Autodesk Inventor part; units mm, degrees
ref_plane "YZ Plane" through (0, 0, 0) normal (1, 0, 0) x (0, 1, 0)
ref_plane "XZ Plane" through (0, 0, 0) normal (0, 1, 0) x (-1, 0, 0)
ref_plane "XY Plane" through (0, 0, 0) normal (0, 0, 1) x (1, 0, 0)
sketch "Sketch1" plane through (0, 0, 0) normal (0, 0, 1) x (1, 0, 0)
  circle A0 centre (0, 0) radius 17.25
  circle A1 centre (0, 0) radius 16.1
  circle A2 centre (0, 0) radius 15
  line L0 (-1, -15.03) -> (1, -15.03)
  line L1 (-1.5, -16.03) -> (1.5, -16.03)
  line L2 (1.5, -16.03) -> (1, -15.03)
  line L3 (-1.5, -16.03) -> (-1, -15.03)
  line L4 (-1, -15.03) -> (-0.9693, -14.9686)
  line L5 (1, -15.03) -> (0.9693, -14.9686)
  line L6 (2.9241, -14.7767) -> (4.856, -14.259)
  line L7 (2.7, -15.872) -> (2.9241, -14.7767)
  line L8 (2.9241, -14.7767) -> (2.9379, -14.7095)
  line L9 (5.5978, -15.0955) -> (4.856, -14.259)
  line L10 (4.856, -14.259) -> (4.8105, -14.2077)
  line L11 (6.649, -13.5163) -> (8.381, -12.5163)
  line L12 (6.7159, -14.6324) -> (6.649, -13.5163)
  line L13 (6.649, -13.5163) -> (6.6449, -13.4479)
  line L14 (9.314, -13.1324) -> (8.381, -12.5163)
  line L15 (8.381, -12.5163) -> (8.3238, -12.4786)
  line L16 (9.9207, -11.3349) -> (11.3349, -9.9207)
  line L17 (10.2742, -12.3956) -> (9.9207, -11.3349)
  line L18 (9.9207, -11.3349) -> (9.899, -11.2699)
  line L19 (12.3956, -10.2742) -> (11.3349, -9.9207)
  line L20 (11.3349, -9.9207) -> (11.2699, -9.899)
  line L21 (12.5163, -8.381) -> (13.5163, -6.649)
  line L22 (13.1324, -9.314) -> (12.5163, -8.381)
  line L23 (12.5163, -8.381) -> (12.4786, -8.3238)
  line L24 (14.6324, -6.7159) -> (13.5163, -6.649)
  line L25 (13.5163, -6.649) -> (13.4479, -6.6449)
  line L26 (14.259, -4.856) -> (14.7767, -2.9241)
  line L27 (15.0955, -5.5978) -> (14.259, -4.856)
  line L28 (14.259, -4.856) -> (14.2077, -4.8105)
  line L29 (15.872, -2.7) -> (14.7767, -2.9241)
  line L30 (14.7767, -2.9241) -> (14.7095, -2.9379)
  line L31 (15.03, -1) -> (15.03, 1)
  line L32 (16.03, -1.5) -> (15.03, -1)
  line L33 (15.03, -1) -> (14.9686, -0.9693)
  line L34 (16.03, 1.5) -> (15.03, 1)
  line L35 (15.03, 1) -> (14.9686, 0.9693)
  line L36 (14.7767, 2.9241) -> (14.259, 4.856)
  line L37 (15.872, 2.7) -> (14.7767, 2.9241)
  line L38 (14.7767, 2.9241) -> (14.7095, 2.9379)
  line L39 (15.0955, 5.5978) -> (14.259, 4.856)
  line L40 (14.259, 4.856) -> (14.2077, 4.8105)
  line L41 (13.5163, 6.649) -> (12.5163, 8.381)
  line L42 (14.6324, 6.7159) -> (13.5163, 6.649)
  line L43 (13.5163, 6.649) -> (13.4479, 6.6449)
  line L44 (13.1324, 9.314) -> (12.5163, 8.381)
  line L45 (12.5163, 8.381) -> (12.4786, 8.3238)
  line L46 (11.3349, 9.9207) -> (9.9207, 11.3349)
  line L47 (12.3956, 10.2742) -> (11.3349, 9.9207)
  line L48 (11.3349, 9.9207) -> (11.2699, 9.899)
  line L49 (10.2742, 12.3956) -> (9.9207, 11.3349)
  line L50 (9.9207, 11.3349) -> (9.899, 11.2699)
  line L51 (8.381, 12.5163) -> (6.649, 13.5163)
  line L52 (9.314, 13.1324) -> (8.381, 12.5163)
  line L53 (8.381, 12.5163) -> (8.3238, 12.4786)
  line L54 (6.7159, 14.6324) -> (6.649, 13.5163)
  line L55 (6.649, 13.5163) -> (6.6449, 13.4479)
  line L56 (4.856, 14.259) -> (2.9241, 14.7767)
  line L57 (5.5978, 15.0955) -> (4.856, 14.259)
  line L58 (4.856, 14.259) -> (4.8105, 14.2077)
  line L59 (2.7, 15.872) -> (2.9241, 14.7767)
  line L60 (2.9241, 14.7767) -> (2.9379, 14.7095)
  line L61 (1, 15.03) -> (-1, 15.03)
  line L62 (1.5, 16.03) -> (1, 15.03)
  line L63 (1, 15.03) -> (0.9693, 14.9686)
  line L64 (-1.5, 16.03) -> (-1, 15.03)
  line L65 (-1, 15.03) -> (-0.9693, 14.9686)
  line L66 (-2.9241, 14.7767) -> (-4.856, 14.259)
  line L67 (-2.7, 15.872) -> (-2.9241, 14.7767)
  line L68 (-2.9241, 14.7767) -> (-2.9379, 14.7095)
  line L69 (-5.5978, 15.0955) -> (-4.856, 14.259)
  line L70 (-4.856, 14.259) -> (-4.8105, 14.2077)
  line L71 (-6.649, 13.5163) -> (-8.381, 12.5163)
  line L72 (-6.7159, 14.6324) -> (-6.649, 13.5163)
  line L73 (-6.649, 13.5163) -> (-6.6449, 13.4479)
  line L74 (-9.314, 13.1324) -> (-8.381, 12.5163)
  line L75 (-8.381, 12.5163) -> (-8.3238, 12.4786)
  line L76 (-9.9207, 11.3349) -> (-11.3349, 9.9207)
  line L77 (-10.2742, 12.3956) -> (-9.9207, 11.3349)
  line L78 (-9.9207, 11.3349) -> (-9.899, 11.2699)
  line L79 (-12.3956, 10.2742) -> (-11.3349, 9.9207)
  line L80 (-11.3349, 9.9207) -> (-11.2699, 9.899)
  line L81 (-12.5163, 8.381) -> (-13.5163, 6.649)
  line L82 (-13.1324, 9.314) -> (-12.5163, 8.381)
  line L83 (-12.5163, 8.381) -> (-12.4786, 8.3238)
  line L84 (-14.6324, 6.7159) -> (-13.5163, 6.649)
  line L85 (-13.5163, 6.649) -> (-13.4479, 6.6449)
  line L86 (-14.259, 4.856) -> (-14.7767, 2.9241)
  line L87 (-15.0955, 5.5978) -> (-14.259, 4.856)
  line L88 (-14.259, 4.856) -> (-14.2077, 4.8105)
  line L89 (-15.872, 2.7) -> (-14.7767, 2.9241)
  line L90 (-14.7767, 2.9241) -> (-14.7095, 2.9379)
  line L91 (-15.03, 1) -> (-15.03, -1)
  line L92 (-16.03, 1.5) -> (-15.03, 1)
  line L93 (-15.03, 1) -> (-14.9686, 0.9693)
  line L94 (-16.03, -1.5) -> (-15.03, -1)
  line L95 (-15.03, -1) -> (-14.9686, -0.9693)
  line L96 (-14.7767, -2.9241) -> (-14.259, -4.856)
  line L97 (-15.872, -2.7) -> (-14.7767, -2.9241)
  line L98 (-14.7767, -2.9241) -> (-14.7095, -2.9379)
  line L99 (-15.0955, -5.5978) -> (-14.259, -4.856)
  line L100 (-14.259, -4.856) -> (-14.2077, -4.8105)
  line L101 (-13.5163, -6.649) -> (-12.5163, -8.381)
  line L102 (-14.6324, -6.7159) -> (-13.5163, -6.649)
  line L103 (-13.5163, -6.649) -> (-13.4479, -6.6449)
  line L104 (-13.1324, -9.314) -> (-12.5163, -8.381)
  line L105 (-12.5163, -8.381) -> (-12.4786, -8.3238)
  line L106 (-11.3349, -9.9207) -> (-9.9207, -11.3349)
  line L107 (-12.3956, -10.2742) -> (-11.3349, -9.9207)
  line L108 (-11.3349, -9.9207) -> (-11.2699, -9.899)
  line L109 (-10.2742, -12.3956) -> (-9.9207, -11.3349)
  line L110 (-9.9207, -11.3349) -> (-9.899, -11.2699)
  line L111 (-8.381, -12.5163) -> (-6.649, -13.5163)
  line L112 (-9.314, -13.1324) -> (-8.381, -12.5163)
  line L113 (-8.381, -12.5163) -> (-8.3238, -12.4786)
  line L114 (-6.7159, -14.6324) -> (-6.649, -13.5163)
  line L115 (-6.649, -13.5163) -> (-6.6449, -13.4479)
  line L116 (-4.856, -14.259) -> (-2.9241, -14.7767)
  line L117 (-5.5978, -15.0955) -> (-4.856, -14.259)
  line L118 (-4.856, -14.259) -> (-4.8105, -14.2077)
  line L119 (-2.7, -15.872) -> (-2.9241, -14.7767)
  line L120 (-2.9241, -14.7767) -> (-2.9379, -14.7095)
  point P0 (0, -16.03)
  point P1 (0, -15.03)
  point P2 (1.5, -16.03)
  point P3 (1.5, -16.03)
  point P4 (3.89, -14.5178)
  point P5 (7.515, -13.0163)
  point P6 (10.6278, -10.6278)
  point P7 (13.0163, -7.515)
  point P8 (14.5178, -3.89)
  point P9 (15.03, 0)
  point P10 (14.5178, 3.89)
  point P11 (13.0163, 7.515)
  point P12 (10.6278, 10.6278)
  point P13 (7.515, 13.0163)
  point P14 (3.89, 14.5178)
  point P15 (0, 15.03)
  point P16 (-3.89, 14.5178)
  point P17 (-7.515, 13.0163)
  point P18 (-10.6278, 10.6278)
  point P19 (-13.0163, 7.515)
  point P20 (-14.5178, 3.89)
  point P21 (-15.03, 0)
  point P22 (-14.5178, -3.89)
  point P23 (-13.0163, -7.515)
  point P24 (-10.6278, -10.6278)
  point P25 (-7.515, -13.0163)
  point P26 (-3.89, -14.5178)
  point P27 (2.7, -15.872)
  point P28 (5.5978, -15.0955)
  point P29 (6.7159, -14.6324)
  point P30 (9.314, -13.1324)
  point P31 (10.2742, -12.3956)
  point P32 (12.3956, -10.2742)
  point P33 (14.6324, -6.7159)
  point P34 (15.872, -2.7)
  point P35 (16.03, -1.5)
  point P36 (16.03, 1.5)
  point P37 (15.872, 2.7)
  point P38 (15.0955, 5.5978)
  point P39 (14.6324, 6.7159)
  point P40 (13.1324, 9.314)
  point P41 (12.3956, 10.2742)
  point P42 (10.2742, 12.3956)
  point P43 (6.7159, 14.6324)
  point P44 (2.7, 15.872)
  point P45 (1.5, 16.03)
  point P46 (-1.5, 16.03)
  point P47 (-5.5978, 15.0955)
  point P48 (-6.7159, 14.6324)
  point P49 (-10.2742, 12.3956)
  point P50 (-12.3956, 10.2742)
  point P51 (-14.6324, 6.7159)
  point P52 (-15.0955, 5.5978)
  point P53 (-15.872, 2.7)
  point P54 (-16.03, -1.5)
  point P55 (-14.6324, -6.7159)
  point P56 (-12.3956, -10.2742)
  point P57 (-10.2742, -12.3956)
  point P58 (-9.314, -13.1324)
  point P59 (-6.7159, -14.6324)
  point P60 (-5.5978, -15.0955)
  point P61 (-2.7, -15.872)
  dimension "d1" = 32.2
  dimension "d0" = 34.5
  dimension "d2" = 30
  dimension "d3" = 2
  dimension "d4" = 3
  dimension "d5" = 1
  dimension "d20" = 360
extrude "Extrusion1" add sketch "Sketch1" along normal blind 15 contours L34 L35 A2 L38 L37 A1 | A1 L29 L30 A2 L33 L32 | L31 L33 A2 L35 | L39 L40 A2 L43 L42 A1 | L38 A2 L40 L36 | A2 | A1 L24 L25 A2 L28 L27 | L26 L28 A2 L30 | L44 L45 A2 L48 L47 A1 | L43 A2 L45 L41 | A1 L19 L20 A2 L23 L22 | L21 L23 A2 L25 | L49 L50 A2 L53 L52 A1 | L48 A2 L50 L46 | A1 L14 L15 A2 L18 L17 | L16 L18 A2 L20 | L54 L55 A2 L58 L57 A1 | L53 A2 L55 L51 | A1 L9 L10 A2 L13 L12 | L11 L13 A2 L15 | L59 L60 A2 L63 L62 A1 | L58 A2 L60 L56 | A1 L2 L5 A2 L8 L7 | L6 L8 A2 L10 | L64 L65 A2 L68 L67 A1 | L63 A2 L65 L61 | A1 L119 L120 A2 L4 L3 | L69 L70 A2 L73 L72 A1 | L68 A2 L70 L66 | A1 L114 L115 A2 L118 L117 | L116 L118 A2 L120 | L74 L75 A2 L78 L77 A1 | L73 A2 L75 L71 | A1 L109 L110 A2 L113 L112 | L111 L113 A2 L115 | L79 L80 A2 L83 L82 A1 | L78 A2 L80 L76 | A1 L104 L105 A2 L108 L107 | L106 L108 A2 L110 | L84 L85 A2 L88 L87 A1 | L83 A2 L85 L81 | A1 L99 L100 A2 L103 L102 | L101 L103 A2 L105 | L89 L90 A2 L93 L92 A1 | L88 A2 L90 L86 | A1 L94 L95 A2 L98 L97 | L96 L98 A2 L100 | L93 A2 L95 L91
sketch "Sketch2" plane through (0, 0, 0) normal (0, 0, -1) x (-1, 0, 0)
  line L0 (12, 6.9282) -> (12, -6.9282)
  line L1 (12, -6.9282) -> (0, -13.8564)
  line L2 (0, -13.8564) -> (-12, -6.9282)
  line L3 (-12, -6.9282) -> (-12, 6.9282)
  line L4 (-12, 6.9282) -> (0, 13.8564)
  line L5 (0, 13.8564) -> (12, 6.9282)
  point P0 (0, 0)
  point P1 (0, 0)
  dimension "d12" = 24
extrude "Extrusion2" add sketch "Sketch2" along normal blind 10
sketch "Sketch3" plane through (0, 0, -10) normal (0, 0, -1) x (-1, 0, 0)
  circle A0 centre (0, 0) radius 7.5
  dimension "d15" = 15
extrude "Extrusion3" [suppressed]
sketch "Sketch4" plane through (0, 0, 0) normal (1, 0, 0) x (0, 1, 0)
  line L0 (20.1089, -13.3141) -> (-23.1689, -13.3141)
  line L1 (-23.1689, -13.3141) -> (-23.1689, 5.9253)
  line L2 (-23.1689, 5.9253) -> (20.1089, 5.9253)
  line L3 (20.1089, 5.9253) -> (20.1089, -13.3141)
  point P0 (0, 0)
extrude "Extrusion4" [suppressed]
properties part number "Nastavek Millard freewheel tool izmerjen trapze"
Check sheet for the modelled part. Datum: model origin and axes. Units: mm. A direction names the side the tool comes from. Give positions to 0.01 mm unless a question says otherwise; leave off trailing zeros. Order: outer loops, then holes, each group sorted by start corner. A loop starts at its lowest first (then second) coordinate and runs counter-clockwise, first axis right, second up. Notation, with made-up numbers: M 41,56.25 L 77,56.25 A13 ccw 77,69.25 Z; hole C -27.75,25.25 d6. An arc over 180 degrees is marked long. Answer as CSV lines item,"result". Start each with the question number.
Item 1: Tool access check on faces 4 (the face through (2.11, -15.96, 7.4)), 5 (the face through (-15.33, -2.81, 7.4)), 6 (the face through (15.537, -1.253, 7.395)), 7 (the face through (-11.87, 10.1, 7.4)), 8 (the face through (8.854, -12.829, 7.395)). Record the directions out of +Z, -Z, +X, -X, +Y, -Y that give a thin tool (end or side, any length) a straight path to the whole face; none if there is none.
Item 2: Thickness scan on line 1 (Y direction, x = 13, z = 13); line 2 (X direction, y = -1, z = -1.75); line 3 (Z direction, x = -2.5, y = -13.5). Record the ranges inside material, lowest first. Write a range as [from, to].
Item 3: Gauge pin test, flat ends, axial feed: P1, Ø3, axis at y = -3, z = -3.5, coming from the +X side; P2, Ø2, axis at x = 9, y = -11, coming from the -Z side; P3, Ø1.5, axis at y = -8, z = 3.5, coming from the +X side; P4, Ø5, axis at x = -3.5, z = 3, coming from the +Y side. Record the tip position at first contact, or that the pin passes through.
Item 4: Cross-section at C-C on y = 2. Enter the section's corners in (x, z).
Item 5: Mould release check, pull along X, two halves, no side actions. Record for faces 1 (the face through (6.683, 14.082, 7.395)), 2 (the face through (-6.683, -14.082, 7.395)), 3 (the face through (7.527, 13.009, 7.395)): +X half, -X half, draft (parallel to the pull), parting line (faces both ways), or undercut.
Item 6: Cross-section at B-B on z = -3.5. Enter the section's corners in (x, y).
Item 7: Cross-section at A-A on y = -3.5. Enter the section's corners in (x, z).
Established:
1,face 4,"+Z, -Z, +X, -Y"
1,face 5,"+Z, -Z, -X"
1,face 6,"+Z, -Z, +X"
1,face 7,"+Z, -Z, +Y"
1,face 8,"+Z, -Z, -Y"
2,line 1,"y = [-9.5, -9.11], [-7.54, 7.54], [9.11, 9.5]"
2,line 2,"x = [-12, 12]"
2,line 3,"z = [0, 15]"
3,P1,"stops at x = 12"
3,P2,"stops at z = 0"
3,P3,"stops at x = 13.17"
3,P4,"stops at y = 16.03"
4,outline,"M -15.98,0 L -12,0 L -12,-10 L 12,-10 L 12,0 L 15.98,0 L 15.98,15 L -15.98,15 Z"
5,face 1,"+X half"
5,face 2,"-X half"
5,face 3,"undercut"
6,outline,"M -12,-6.93 L 0,-13.86 L 12,-6.93 L 12,6.93 L 0,13.86 L -12,6.93 Z"
7,outline,"M -14.62,0 L -12,0 L -12,-10 L 12,-10 L 12,0 L 14.62,0 L 14.62,15 L -14.62,15 Z"
